from build123d import *

# Parameters (mm, degrees)
EXTRUDE_2_DEPTH     = 10
SCALE_2_SCALE       = 3
SKETCH_5_W          = 154.243752884
SKETCH_5_H          = 20
CUT_EXTRUDE_1_DEPTH = 113.5
SKETCH_6_R          = 5
CUT_EXTRUDE_2_DEPTH = 113.5


with BuildPart() as part:
    # 草图4 → 凸台-拉伸2 (new body)
    with BuildSketch(Plane(origin=(0, 0, 0), x_dir=(1, 0, 0), z_dir=(0, 1, 0))):
        with BuildLine():
            ThreePointArc((-13.678571429, 2.982730909), (-12.124355653, 7), (-9.422406454, 10.35462489))
            ThreePointArc((-9.422406454, 10.35462489), (-9.513861615, 10.487132461), (-9.598076211, 10.624355653))
            Line((-9.598076211, 10.624355653), (-15.762896757, 21.302138058))
            ThreePointArc((-15.762896757, 21.302138058), (-17.464105133, 19.93125766), (-19.046604272, 18.424897983))
            ThreePointArc((-19.046604272, 18.424897983), (-18.7975102, 17.224138351), (-18.71396178, 16.000663294))
            ThreePointArc((-18.71396178, 16.000663294), (-20.603825728, 10.482877024), (-25.479731852, 7.282394164))
            ThreePointArc((-25.479731852, 7.282394164), (-25.993028029, 5.158729869), (-26.329641091, 3))
            Line((-26.329641091, 3), (-14, 3))
            ThreePointArc((-14, 3), (-13.839053931, 2.995679616), (-13.678571429, 2.982730909))
        make_face()
        with BuildLine():
            ThreePointArc((13.678571429, -2.982730909), (11.767928573, -2.004459314), (11, 0))
            Line((11, 0), (0, 0))
            Line((0, 0), (12.124355653, 7))
            ThreePointArc((12.124355653, 7), (10.903170014, 8.781849671), (9.422406454, 10.35462489))
            ThreePointArc((9.422406454, 10.35462489), (5.5, 9.526279442), (4.256164975, 13.337355799))
            ThreePointArc((4.256164975, 13.337355799), (0, 14), (-4.256164975, 13.337355799))
            ThreePointArc((-4.256164975, 13.337355799), (-4.064739784, 12.744232626), (-4, 12.124355653))
            ThreePointArc((-4, 12.124355653), (-6.069199098, 9.272407252), (-9.422406454, 10.35462489))
            ThreePointArc((-9.422406454, 10.35462489), (-12.124355653, 7), (-13.678571429, 2.982730909))
            ThreePointArc((-13.678571429, 2.982730909), (-11.767928573, 2.004459314), (-11, 0))
            ThreePointArc((-11, 0), (-11.767928573, -2.004459314), (-13.678571429, -2.982730909))
            ThreePointArc((-13.678571429, -2.982730909), (-12.124355653, -7), (-9.422406454, -10.35462489))
            ThreePointArc((-9.422406454, -10.35462489), (-6.069199098, -9.272407252), (-4, -12.124355653))
            ThreePointArc((-4, -12.124355653), (-4.064739784, -12.744232626), (-4.256164975, -13.337355799))
            ThreePointArc((-4.256164975, -13.337355799), (0, -14), (4.256164975, -13.337355799))
            ThreePointArc((4.256164975, -13.337355799), (5.5, -9.526279442), (9.422406454, -10.35462489))
            ThreePointArc((9.422406454, -10.35462489), (12.124355653, -7), (13.678571429, -2.982730909))
        make_face()
        with BuildLine():
            ThreePointArc((-4.256164975, 13.337355799), (0, 14), (4.256164975, 13.337355799))
            ThreePointArc((4.256164975, 13.337355799), (4.325192316, 13.482812077), (4.401923789, 13.624355653))
            Line((4.401923789, 13.624355653), (10.566744334, 24.302138058))
            ThreePointArc((10.566744334, 24.302138058), (8.528922897, 25.089987529), (6.433127579, 25.707292147))
            ThreePointArc((6.433127579, 25.707292147), (0, 23.001326589), (-6.433127579, 25.707292147))
            ThreePointArc((-6.433127579, 25.707292147), (-8.528922897, 25.089987529), (-10.566744334, 24.302138058))
            Line((-10.566744334, 24.302138058), (-4.401923789, 13.624355653))
            ThreePointArc((-4.401923789, 13.624355653), (-4.325192316, 13.482812077), (-4.256164975, 13.337355799))
        make_face()
        with BuildLine():
            ThreePointArc((9.422406454, 10.35462489), (10.903170014, 8.781849671), (12.124355653, 7))
            Line((12.124355653, 7), (19.919733146, 11.500663294))
            ThreePointArc((19.919733146, 11.500663294), (18.784672274, 14.874701965), (19.046604272, 18.424897983))
            ThreePointArc((19.046604272, 18.424897983), (17.464105133, 19.93125766), (15.762896757, 21.302138058))
            Line((15.762896757, 21.302138058), (9.598076211, 10.624355653))
            ThreePointArc((9.598076211, 10.624355653), (9.513861615, 10.487132461), (9.422406454, 10.35462489))
        make_face()
        with BuildLine():
            ThreePointArc((12.124355653, 7), (13.056889914, 5.051497379), (13.678571429, 2.982730909))
            ThreePointArc((13.678571429, 2.982730909), (13.839053931, 2.995679616), (14, 3))
            Line((14, 3), (26.329641091, 3))
            ThreePointArc((26.329641091, 3), (25.993028029, 5.158729869), (25.479731852, 7.282394164))
            ThreePointArc((25.479731852, 7.282394164), (22.274205913, 8.830652409), (19.919733146, 11.500663294))
            Line((19.919733146, 11.500663294), (12.124355653, 7))
        make_face()
        with BuildLine():
            ThreePointArc((14, -3), (13.839053931, -2.995679616), (13.678571429, -2.982730909))
            ThreePointArc((13.678571429, -2.982730909), (12.124355653, -7), (9.422406454, -10.35462489))
            ThreePointArc((9.422406454, -10.35462489), (9.513861615, -10.487132461), (9.598076211, -10.624355653))
            Line((9.598076211, -10.624355653), (15.762896757, -21.302138058))
            ThreePointArc((15.762896757, -21.302138058), (17.464105133, -19.93125766), (19.046604272, -18.424897983))
            ThreePointArc((19.046604272, -18.424897983), (19.919733146, -11.500663294), (25.479731852, -7.282394164))
            ThreePointArc((25.479731852, -7.282394164), (25.993028029, -5.158729869), (26.329641091, -3))
            Line((26.329641091, -3), (14, -3))
        make_face()
        with BuildLine():
            ThreePointArc((4.401923789, -13.624355653), (4.325192316, -13.482812077), (4.256164975, -13.337355799))
            ThreePointArc((4.256164975, -13.337355799), (0, -14), (-4.256164975, -13.337355799))
            ThreePointArc((-4.256164975, -13.337355799), (-4.325192316, -13.482812077), (-4.401923789, -13.624355653))
            Line((-4.401923789, -13.624355653), (-10.566744334, -24.302138058))
            ThreePointArc((-10.566744334, -24.302138058), (-8.528922897, -25.089987529), (-6.433127579, -25.707292147))
            ThreePointArc((-6.433127579, -25.707292147), (0, -23.001326589), (6.433127579, -25.707292147))
            ThreePointArc((6.433127579, -25.707292147), (8.528922897, -25.089987529), (10.566744334, -24.302138058))
            Line((10.566744334, -24.302138058), (4.401923789, -13.624355653))
        make_face()
        with BuildLine():
            ThreePointArc((-9.598076211, -10.624355653), (-9.513861615, -10.487132461), (-9.422406454, -10.35462489))
            ThreePointArc((-9.422406454, -10.35462489), (-12.124355653, -7), (-13.678571429, -2.982730909))
            ThreePointArc((-13.678571429, -2.982730909), (-13.839053931, -2.995679616), (-14, -3))
            Line((-14, -3), (-26.329641091, -3))
            ThreePointArc((-26.329641091, -3), (-25.993028029, -5.158729869), (-25.479731852, -7.282394164))
            ThreePointArc((-25.479731852, -7.282394164), (-20.603825728, -10.482877024), (-18.71396178, -16.000663294))
            ThreePointArc((-18.71396178, -16.000663294), (-18.7975102, -17.224138351), (-19.046604272, -18.424897983))
            ThreePointArc((-19.046604272, -18.424897983), (-17.464105133, -19.93125766), (-15.762896757, -21.302138058))
            Line((-15.762896757, -21.302138058), (-9.598076211, -10.624355653))
        make_face()
        with BuildLine():
            Line((0, 0), (11, 0))
            ThreePointArc((11, 0), (11.767928573, 2.004459314), (13.678571429, 2.982730909))
            ThreePointArc((13.678571429, 2.982730909), (13.056889914, 5.051497379), (12.124355653, 7))
            Line((12.124355653, 7), (0, 0))
        make_face()
    extrude(amount=EXTRUDE_2_DEPTH)


with BuildPart() as part_1:
    # 缩放比例2: scaled about (0, 5, 0)
    add(part.part.scale(SCALE_2_SCALE).moved(Location((0, -10, 0))))

    # 草图5 → 切除-拉伸1 (cut, symmetric)
    with BuildSketch(Plane(origin=(0, 0, 0), x_dir=(0, 0, -1), z_dir=(1, 0, 0))):
        with Locations((0, 10)):
            Rectangle(SKETCH_5_W, SKETCH_5_H)
    extrude(amount=CUT_EXTRUDE_1_DEPTH, both=True, mode=Mode.SUBTRACT)

    # 草图6 → 切除-拉伸2 (cut, symmetric)
    with BuildSketch(Plane.XZ.offset(10)):
        with Locations(Location((0, 0, 0), (0, 0, 270))):
            Circle(SKETCH_6_R)
    extrude(amount=CUT_EXTRUDE_2_DEPTH, both=True, mode=Mode.SUBTRACT)


solid = part_1.part
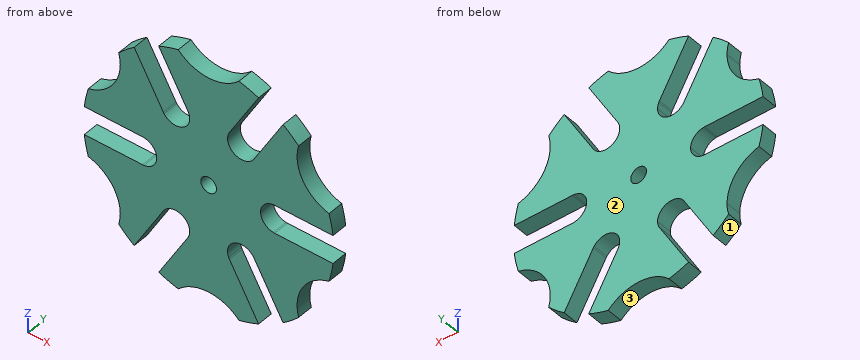
Design review of the part built by this model. Coordinates are the model's own, in mm. Face numbers are marked on the shaded views. Coordinates: 2 decimals unless noted, no trailing zeros. Write each loop counter-clockwise with the first axis right and the second up, starting at its lowest first coordinate (ties: lowest second). Pieces come first, ordered by that corner, then holes. Notation, with made-up numbers: (80.25, 89.25) - (123.25, 89.25) arc R19 cw to (123.25, 119.25) - close; hole circle Ø11 at (3.5, 35.5). An arc over 180 degrees is marked (long way). One line per item, written item: value.
1) Insertion check: pin 1 (3 mm diameter, centred on x = 52.5, y = -7, fed in from +Z); pin 2 (5 mm diameter, centred on y = -1.5, z = 54.5, fed in from -X); pin 3 (5 mm diameter, centred on x = -11.5, y = -7.5, fed in from -Z); pin 4 (6 mm diameter, centred on x = 0, z = 0, fed in from -Y). Each pin has a flat end and moves straight along its axis. Give the tip position at first contact, or say it passes through.
Answer sheet:
pin 1: stops at z = 60.99
pin 2: stops at x = -57.14
pin 3: stops at z = -72.92
pin 4: passes through
2) Add section B-B (z = 44.5). State the section outline as (x, y) points.
Answer sheet:
outline: (-56.37, -10) - (-36.08, -10) - (-36.08, 0) - (-56.37, 0) - close; (-15.3, -10) - (15.3, -10) - (15.3, 0) - (-15.3, 0) - close; (36.08, -10) - (56.37, -10) - (56.37, 0) - (36.08, 0) - close
3) Add section A-A (x = 0). State the section outline as (y, z) points.
Answer sheet:
outline: (-10, -69) - (0, -69) - (0, -5) - (-10, -5) - close; (-10, 5) - (0, 5) - (0, 69) - (-10, 69) - close
4) Mouldability with a two-part tool opening along X and no side actions: class the marked faces 1, 2 and 3 as +X half, -X half, draft (parallel to the pull), parting line (faces both ways), or undercut.
Answer sheet:
face 1: -X half
face 2: draft
face 3: undercut
5) To check wall thickness, follow probe 1 along X at (y, z) = (-6.5, 45.5); probe 2 along X at (y, z) = (-2, -52); probe 3 along Z at (x, y) = (-13, -9.25). State the ranges of each line that lie inside material, in increasing order.
Answer sheet:
probe 1: x = -56.26 to -36.66, -15.88 to 15.88, 36.66 to 56.26
probe 2: x = -56.44 to -40.41, -19.63 to 19.63, 40.41 to 56.44
probe 3: z = -72.34 to -40.5, -32.25 to 32.25, 40.5 to 72.34
6) Add section C-C (x = 68). State the section outline as (y, z) points, plus the area to 3 significant figures.
Answer sheet:
outline: (-10, -25.65) - (0, -25.65) - (0, -9) - (-10, -9) - close; (-10, 9) - (0, 9) - (0, 25.65) - (-10, 25.65) - close
area: 333 mm2
